Could you check a few things on this model? Use its own coordinates, in mm. Coordinates: 2 decimals unless noted, no trailing zeros. One line per question, with ' | ' between items.
from build123d import *

# Parameters (mm, degrees)
SKETCH1_W                                 = 762
SKETCH1_H                                 = 266.7
BOSS_EXTRUDE1_DEPTH                       = 19.05
CBORE_FOR_5_16_HEX_HEAD_BOLT1_D           = 8.4328
CBORE_FOR_5_16_HEX_HEAD_BOLT1_CBORE_D     = 20.6375
CBORE_FOR_5_16_HEX_HEAD_BOLT1_CBORE_DEPTH = 9.144
F_1_4_CLEARANCE_HOLE1_D                   = 7.14248


with BuildPart() as part:
    # Sketch1 → Boss-Extrude1 (new body)
    with BuildSketch(Plane(origin=(0, 0, 0), x_dir=(1, 0, 0), z_dir=(0, 1, 0))):
        Rectangle(SKETCH1_W, SKETCH1_H)
    extrude(amount=BOSS_EXTRUDE1_DEPTH)

    # CBORE for 5/16 Hex Head Bolt1 (through all)
    with Locations(Plane(origin=(0, 19.05, 0), x_dir=(1, 0, 0), z_dir=(0, 1, 0))):
        with Locations((-330.2, 114.3), (-292.1, 114.3), (-254, 76.2), (-254, 38.1), (-215.9, 114.3), (-177.8, 114.3), (76.2, 114.3), (114.3, 114.3), (152.4, 76.2), (152.4, 38.1), (190.5, 114.3), (228.6, 114.3), (228.6, -114.3), (190.5, -114.3), (152.4, -38.1), (152.4, -76.2), (114.3, -114.3), (76.2, -114.3), (-177.8, -114.3), (-215.9, -114.3), (-254, -38.1), (-254, -76.2), (-292.1, -114.3), (-330.2, -114.3)):
            CounterBoreHole(CBORE_FOR_5_16_HEX_HEAD_BOLT1_D / 2, CBORE_FOR_5_16_HEX_HEAD_BOLT1_CBORE_D / 2, CBORE_FOR_5_16_HEX_HEAD_BOLT1_CBORE_DEPTH)

    # 1/4 Clearance Hole1 (through all)
    with Locations(Plane(origin=(0, 19.05, 0), x_dir=(1, 0, 0), z_dir=(0, 1, 0))):
        with Locations((-330.2, 0), (-279.4, 0), (-228.6, 0), (-177.8, 0), (-127, 0), (-76.2, 0), (-25.4, 0), (25.4, 0), (76.2, 0), (127, 0), (177.8, 0), (228.6, 0), (361.95, 114.3), (336.55, 114.3), (311.15, 114.3), (285.75, 114.3), (336.55, 88.9), (311.15, 88.9), (285.75, 88.9), (336.55, 63.5), (311.15, 63.5), (285.75, 63.5), (336.55, 38.1), (311.15, 38.1), (285.75, 38.1), (336.55, -38.1), (311.15, -38.1), (285.75, -38.1), (336.55, -63.5), (311.15, -63.5), (285.75, -63.5), (336.55, -88.9), (311.15, -88.9), (285.75, -88.9), (336.55, -114.3), (311.15, -114.3), (285.75, -114.3), (361.95, 88.9), (361.95, 63.5), (361.95, 38.1), (361.95, -38.1), (361.95, -63.5), (361.95, -88.9), (361.95, -114.3), (361.95, 0), (336.55, 0), (311.15, 0), (285.75, 0)):
            Hole(F_1_4_CLEARANCE_HOLE1_D / 2)


solid = part.part
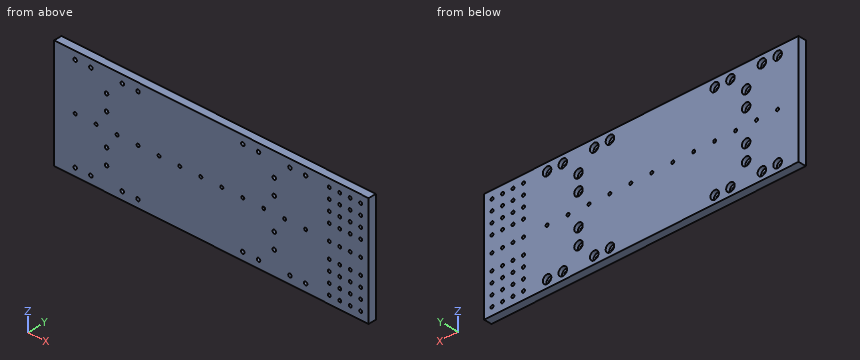
1) If we section it at A-A on y = 13.25: Give the number of separate pieces and of enclosed holes in the cut face, and give its area (3 significant figures).
Data:
separate pieces: 1 | enclosed holes: 72 | area: 193,000 mm²
2) I'm going to push flat-ended pins straight in: pin 1 Ø10.5 at (x, z) = (-293.5, -111.5) entering from +Y; pin 2 Ø4.5 at (x, z) = (361.95, 63.5) entering from +Y. Where does each tip first touch, or does it pass through?
Data:
pin 1: y = 9.91 | pin 2: through
3) I need wall thicknesses on line 1 along X through (y, z) = (8.75, -89); line 2 along Z through (x, y) = (152.4, 13); line 3 along Z through (x, y) = (228.6, 6.5). Which ranges of each line are inside material? Lowest first, please. Write a range as from..to.
Data:
line 1: -381..282.18, 289.32..307.58, 314.72..332.98, 340.12..358.38, 365.52..381 | line 2: -133.35..-86.52, -65.88..-48.42, -27.78..27.78, 48.42..65.88, 86.52..133.35 | line 3: -133.35..-118.52, -110.08..-3.57, 3.57..110.08, 118.52..133.35
